```python
from build123d import *

# Parameters (mm, degrees)
F0_W     = 36
F0_H     = 18
F1_DEPTH = 3
F2_W     = 30.1
F2_H     = 12.92
F3_DEPTH = 2
F4_W     = 8
F4_H     = 8
F5_DEPTH = 3.001
F6_R     = 2
F7_R     = 1
F8_DEPTH = 2


with BuildPart() as f1:
    # F0 (on Top) → F1 (new body)
    with BuildSketch(Plane.XY):
        Rectangle(F0_W, F0_H)
    extrude(amount=F1_DEPTH)

    # F2 (on face) → F3 (cut)
    with BuildSketch(Plane.XY.offset(3)):
        Rectangle(F2_W, F2_H)
    extrude(amount=-F3_DEPTH, mode=Mode.SUBTRACT)

    # F4 (on face) → F5 (cut, through all)
    with BuildSketch(Plane(origin=(0, 0, 0), x_dir=(1, 0, 0), z_dir=(0, 0, -1))):
        Rectangle(F4_W, F4_H)
    extrude(amount=-F5_DEPTH, mode=Mode.SUBTRACT)

    # F6
    f6_edges = [f1.edges().sort_by_distance(p)[0] for p in [
        (-18, -9, 1.5),
        (-18, 9, 1.5),
        (18, -9, 1.5),
        (18, 9, 1.5),
    ]]
    fillet(f6_edges, radius=F6_R)

    # F7 (on face) → F8 (cut)
    with BuildSketch(Plane.XY.offset(3)):
        with Locations((-15.05, 6.46)):
            Circle(F7_R)
        with Locations((-15.05, -6.46)):
            Circle(F7_R)
        with Locations((15.05, 6.46)):
            Circle(F7_R)
        with Locations((15.05, -6.46)):
            Circle(F7_R)
    extrude(amount=-F8_DEPTH, mode=Mode.SUBTRACT)


solid = f1.part
```
Input: part model. Units: mm. Frame: model coordinates. A direction names the side the tool comes from. Give positions to 0.01 mm unless a question says otherwise; leave off trailing zeros. Loops run counter-clockwise (first coordinate to the right, second up) from the corner with the lowest first, then second, coordinate; pieces in that order, holes last.
1) Section query B-B on z = 0.45. Return the cut outline in (x, y), and give its area (3 significant figures).
A:
outline: (-18, -7) arc R2 ccw to (-16, -9) - (16, -9) arc R2 ccw to (18, -7) - (18, 7) arc R2 ccw to (16, 9) - (-16, 9) arc R2 ccw to (-18, 7) - close; hole (-4, -4) - (4, -4) - (4, 4) - (-4, 4) - close
area: 581 mm2
2) Section query D-D on y = 4.5. Return the cut outline in (x, z).
A:
outline: (-18, 0) - (18, 0) - (18, 3) - (15.05, 3) - (15.05, 1) - (-15.05, 1) - (-15.05, 3) - (-18, 3) - close
3) Line query: L1, parallel to X at y = -1.25, z = 1.5; L2, parallel to X at y = -3, z = 0.3; L3, parallel to Y at x = -7, z = 1.6. Output: solid intervals per line, ascending.
A:
L1: x = -18 to -15.05, 15.05 to 18
L2: x = -18 to -4, 4 to 18
L3: y = -9 to -6.46, 6.46 to 9
4) Reachability of faces 1 (the cylindrical face through (15.733, -7.19, 2.014)), 2 (the flat face through (-4, 0.1, 0.5)), 3 (the cylindrical face through (17.4, 8.43, 1.52)) from +Z, -Z, +X, -X, +Y, -Y: full face, straight path, thin tool, end or side. Return the list, or none.
A:
face 1: +Z
face 2: +Z, -Z
face 3: +Z, -Z, +X, +Y
5) Section query C-C on y = -0.25. Return the cut outline in (x, z).
A:
outline: (-18, 0) - (-4, 0) - (-4, 1) - (-15.05, 1) - (-15.05, 3) - (-18, 3) - close; (4, 0) - (18, 0) - (18, 3) - (15.05, 3) - (15.05, 1) - (4, 1) - close
6) Contact query for a flat-ended pin moving along its axis: pin 1 (1.6 mm diameter, centred on x = 15.05, y = 6.46, fed in from +Z). Output: stop coordinate, or through.
A:
pin 1: stops at z = 1
7) Mould query, pull axis X, two halves, no side actions, for faces 4 (the flat face through (-18, 0, 1)), 5 (the flat face through (0, 9, 1)), 6 (the flat face through (18, 0, 1)), 7 (the cylindrical face through (-15.733, 7.19, 2.014)). Classes: released by +X, released by -X, zero draft, split by the parting line, or undercut.
A:
face 4: released by -X
face 5: zero draft
face 6: released by +X
face 7: undercut
8) Section query A-A on x = -0.5. Return the cut outline in (y, z), and give its area (3 significant figures).
A:
outline: (-9, 0) - (-4, 0) - (-4, 1) - (-6.46, 1) - (-6.46, 3) - (-9, 3) - close; (4, 0) - (9, 0) - (9, 3) - (6.46, 3) - (6.46, 1) - (4, 1) - close
area: 20.2 mm2
